```python
from build123d import *

# Parameters (mm, degrees)
SKETCH1_R           = 1.75
BOSS_EXTRUDE1_DEPTH = 2


with BuildPart() as part:
    # Sketch1 → Boss-Extrude1 (new body)
    with BuildSketch(Plane.XY):
        with BuildLine():
            Line((4.472135955, 0.5), (12.123157342, 0.5))
            ThreePointArc((12.123157342, 0.5), (12.486721612, 0.568430882), (12.800527834, 0.764357957))
            Line((12.800527834, 0.764357957), (18.199472166, 5.735642043))
            ThreePointArc((18.199472166, 5.735642043), (18.513278388, 5.931569118), (18.876842658, 6))
            Line((18.876842658, 6), (22, 6))
            ThreePointArc((22, 6), (22.353553391, 6.146446609), (22.5, 6.5))
            Line((22.5, 6.5), (22.5, 10))
            Line((22.5, 10), (25.5, 10))
            Line((25.5, 10), (25.5, 9))
            Line((25.5, 9), (45.5, 9))
            Line((45.5, 9), (45.5, 10))
            Line((45.5, 10), (48.5, 10))
            Line((48.5, 10), (48.5, 8.397324532))
            ThreePointArc((48.5, 8.397324532), (48.366025404, 7.897324532), (48, 7.531299129))
            Line((48, 7.531299129), (25.723862599, -5.329834796))
            Line((25.723862599, -5.329834796), (18.732975398, -9.366025404))
            ThreePointArc((18.732975398, -9.366025404), (18.491794443, -9.465925826), (18.232975398, -9.5))
            Line((18.232975398, -9.5), (12.871682623, -9.5))
            ThreePointArc((12.871682623, -9.5), (12.48899919, -9.423879533), (12.164575841, -9.207106781))
            Line((12.164575841, -9.207106781), (9.500810677, -6.543341617))
            ThreePointArc((9.500810677, -6.543341617), (9.176387328, -6.326568865), (8.793703896, -6.250448398))
            Line((8.793703896, -6.250448398), (2.16466196, -6.250448398))
            ThreePointArc((2.16466196, -6.250448398), (1.781978528, -6.17432793), (1.457555179, -5.957555179))
            Line((1.457555179, -5.957555179), (0, -4.5))
            ThreePointArc((0, -4.5), (-3.354101966, 3), (4.472135955, 0.5))
        make_face()
        Circle(SKETCH1_R, mode=Mode.SUBTRACT)
        with BuildLine():
            Line((27.801871392, 6.5), (39.347712108, 6.5))
            ThreePointArc((39.347712108, 6.5), (39.830675021, 6.129409523), (39.597712108, 5.566987298))
            Line((39.597712108, 5.566987298), (33.04143505, 1.781718974))
            ThreePointArc((33.04143505, 1.781718974), (32.475981159, 1.649888783), (31.932592907, 1.854452979))
            Line((31.932592907, 1.854452979), (27.047958678, 5.6033543))
            ThreePointArc((27.047958678, 5.6033543), (26.878922862, 6.160743818), (27.35237975, 6.5))
            Line((27.35237975, 6.5), (27.801871392, 6.5))
        make_face(mode=Mode.SUBTRACT)
        with BuildLine():
            Line((29.525805665, 0.550207783), (26.468512346, 2.8966457))
            ThreePointArc((26.468512346, 2.8966457), (26.324835093, 2.973456888), (26.164091274, 3))
            Line((26.164091274, 3), (23.793857984, 3))
            ThreePointArc((23.793857984, 3), (23.440304593, 2.853553391), (23.293857984, 2.5))
            Line((23.293857984, 2.5), (23.293857984, -2.980021865))
            ThreePointArc((23.293857984, -2.980021865), (23.543857984, -3.413034567), (24.043857984, -3.413034567))
            Line((24.043857984, -3.413034567), (29.471384593, -0.279450618))
            ThreePointArc((29.471384593, -0.279450618), (29.72031239, 0.120835138), (29.525805665, 0.550207783))
        make_face(mode=Mode.SUBTRACT)
        Polygon((14.565442371, -1.000856688), (14.434557629, -5.999143312), (16.433872279, -6.051497209), (16.564757021, -1.053210584), align=None, mode=Mode.SUBTRACT)
    extrude(amount=BOSS_EXTRUDE1_DEPTH)


solid = part.part
```
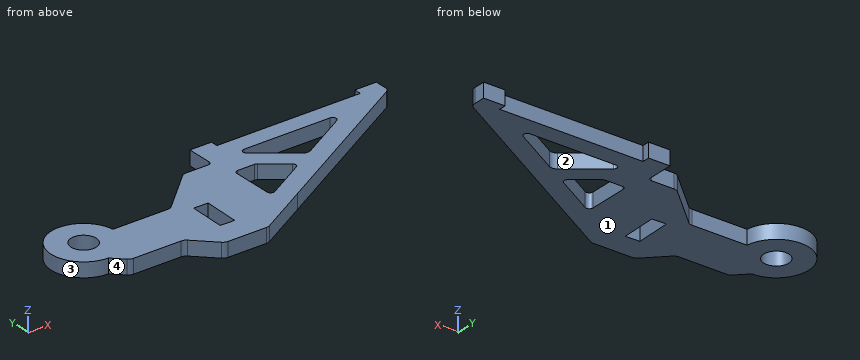
The listing builds one solid part. Answer for the finished solid, in the listing's coordinates (mm). Face numbers are marked on the shaded views. Coordinates: 2 decimals unless noted, no trailing zeros. Loops run counter-clockwise (first coordinate to the right, second up) from the corner with the lowest first, then second, coordinate; pieces in that order, holes last. Notation, with made-up numbers: (45.5, 21) - (75.5, 21) arc R8 cw to (75.5, 31) - close; hole circle Ø7 at (2, 1.25). An arc over 180 degrees is marked (long way). Use a Markdown table: item, result. Add a question column.
1) The part is cut by section A-A, the plane x = 28.5. Give the vertices of the cut face in (y, z).
2) The part is cut by section B-B, the plane x = -0.5. Give the vertices of the cut face in (y, z).
3) The part is cut by section C-C, the plane y = -2.5. Give the vertices of the cut face in (x, z).
4) The mould has two halves that part along X. Classify the marked faces 1, 2, 3 and 4: released by +X, released by -X, zero draft, split by the parting line, or undercut.
5) Given pin 1 (4.5 mm diameter, centred on x = 0, y = 0, fed in from +Z); pin 2 (0.6 mm diameter, centred on x = 8.5, z = 1.5, fed in from +Y); pin 3 (1 mm diameter, centred on x = 5.5, z = 1, fed in from -Y); pin 4 (1.1 mm diameter, centred on y = 9.5, z = 0.5, fed in from -X), each flat-ended and moving along its own axis, determine where each tip first touches the part or whether it passes through.
6) The part is cut by section D-D, the plane z = 0.3. State how many separate pieces and enclosed holes the cut face has, and give its area (3 significant figures).
7) Find the intervals of material crossed by line 1 (Y direction, x = 0, z = 1.25); line 2 (X direction, y = -1.5, z = 0.4); line 3 (Y direction, x = 4.5, z = 0.4), in increasing order.
Here are the results:
| question | item | result |
|---|---|---|
| 1 | outline | (-3.73, 0) - (-0.84, 0) - (-0.84, 2) - (-3.73, 2) - close; (1.34, 0) - (4.49, 0) - (4.49, 2) - (1.34, 2) - close; (6.5, 0) - (9, 0) - (9, 2) - (6.5, 2) - close |
| 2 | outline | (-4.47, 0) - (-1.68, 0) - (-1.68, 2) - (-4.47, 2) - close; (1.68, 0) - (4.47, 0) - (4.47, 2) - (1.68, 2) - close |
| 3 | outline | (-3.74, 0) - (14.53, 0) - (14.53, 2) - (-3.74, 2) - close; (16.53, 0) - (23.29, 0) - (23.29, 2) - (16.53, 2) - close; (25.63, 0) - (30.63, 0) - (30.63, 2) - (25.63, 2) - close |
| 4 | face 1 | zero draft |
| 4 | face 2 | undercut |
| 4 | face 3 | undercut |
| 4 | face 4 | released by -X |
| 5 | pin 1 | stops at z = 2 |
| 5 | pin 2 | stops at y = 0.5 |
| 5 | pin 3 | stops at y = -6.25 |
| 5 | pin 4 | stops at x = 22.5 |
| 6 | separate pieces | 1 |
| 6 | enclosed holes | 4 |
| 6 | area | 415 mm^2 |
| 7 | line 1 | y = -4.5 to -1.75, 1.75 to 4.5 |
| 7 | line 2 | x = -4.24 to -0.9, 0.9 to 14.55, 16.55 to 23.29, 27.36 to 32.36 |
| 7 | line 3 | y = -6.25 to 0.5 |
